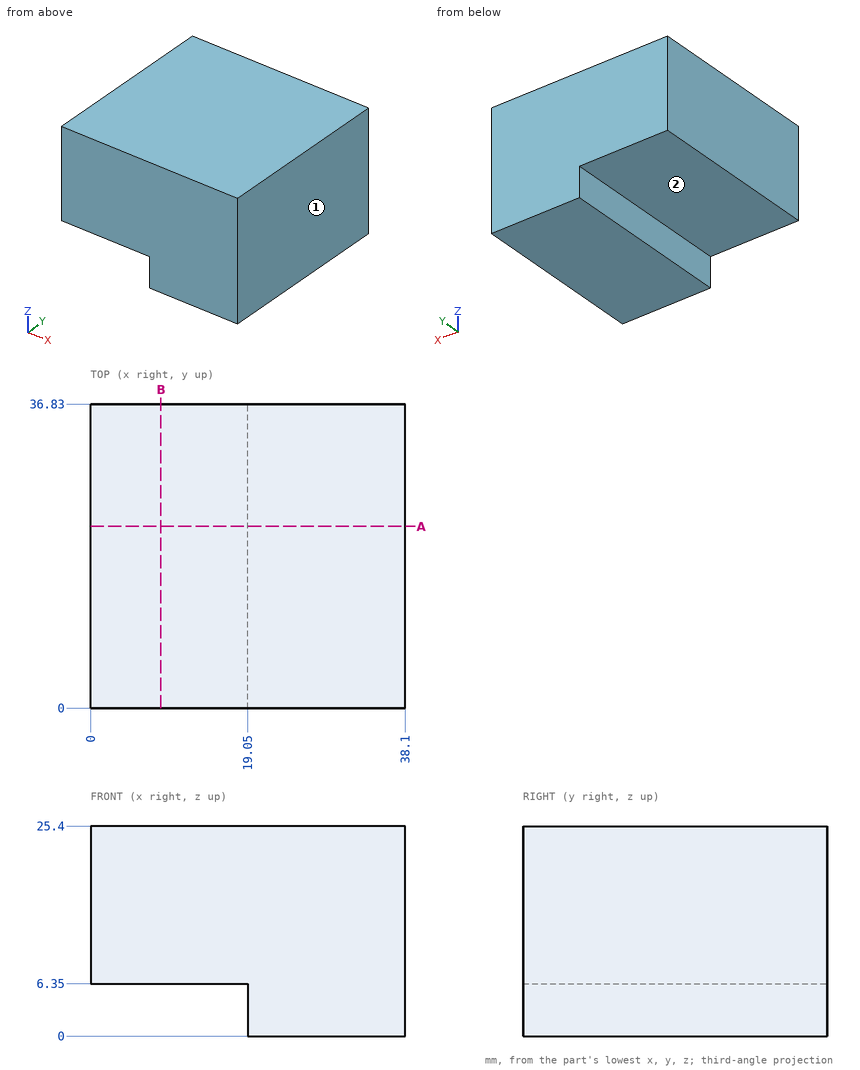
Job drawing, mm, ordinate dimensions from the low corner. One solid piece. A direction names the side the tool comes from. Round coordinates to 2 decimals unless told otherwise and drop trailing zeros. Write each loop counter-clockwise with the first axis right and the second up, starting at its lowest first coordinate (ties: lowest second). Pieces come first, ordered by that corner, then holes. Notation, with made-up numbers: (-28, 40.5) -> (-10, 40.5) arc R22 ccw to (-10, 78.5) -> close; hole circle Ø1 at (35, -30.5). An arc over 180 degrees is marked (long way). Answer as a JSON object with one key per item and string values.
(1) Band-saw the part on B-B, the plane x = 8.5. List the corners of the cut face in (y, z).
Reported:
{"outline": "(0, 6.35) -> (36.83, 6.35) -> (36.83, 25.4) -> (0, 25.4) -> close"}
(2) Probe probe 1 along Z at (x, y) = (5, 21.5); probe 2 along X at (y, z) = (22, 3.5). List the from-to ranges inside material, lowest first. Write a range as [from, to].
Reported:
{"probe 1": "z = [6.35, 25.4]", "probe 2": "x = [19.05, 38.1]"}
(3) Which spindle directions (+Z, -Z, +X, -X, +Y, -Y) get a long thin tool onto all of the face, cutting with end or side? Do the marked faces 1 and 2. Say none if no direction does.
Reported:
{"face 1": "+Z, -Z, +X, +Y, -Y", "face 2": "-Z, -X, +Y, -Y"}
(4) Band-saw the part on A-A, the plane y = 22. List the corners of the cut face in (x, z), then the cut area to 3 significant figures.
Reported:
{"outline": "(0, 6.35) -> (19.05, 6.35) -> (19.05, 0) -> (38.1, 0) -> (38.1, 25.4) -> (0, 25.4) -> close", "area": "847 mm^2"}
(5) Pin check, flat tips, straight feed: P1, Ø2, axis at x = 29, z = 19.5, coming from the -Y side; P2, Ø8, axis at x = 11.5, y = 27.5, coming from the -Z side; P3, Ø1.9, axis at y = 23, z = 3.5, coming from the -X side. Stop position of each tip, or through.
Reported:
{"P1": "stops at y = 0", "P2": "stops at z = 6.35", "P3": "stops at x = 19.05"}
